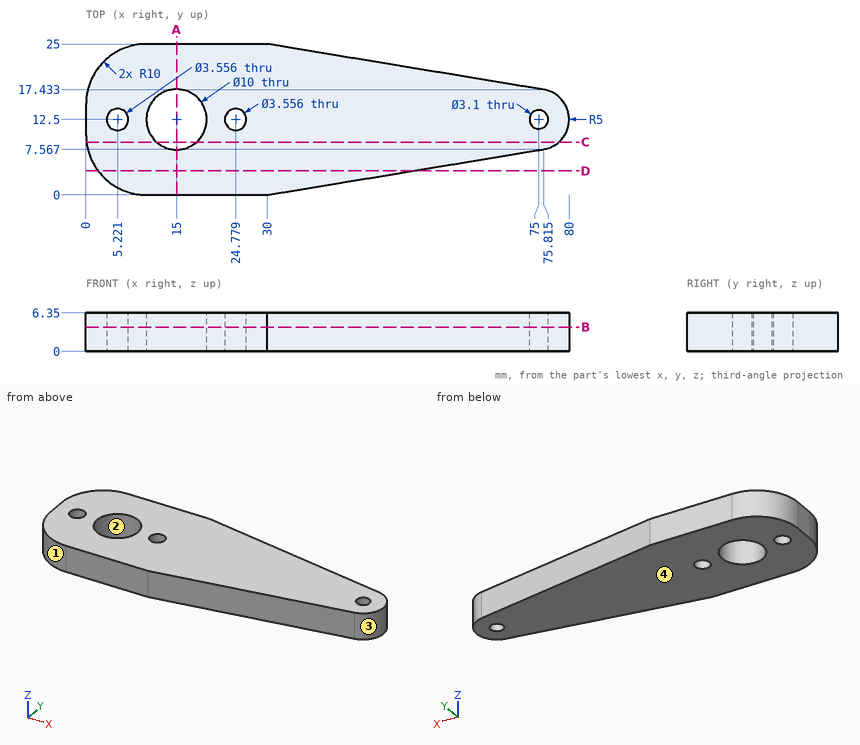
Here's the drawing with two shaded views (mm, measured from the low corner). I have some questions. Coordinates: 2 decimals unless noted, no trailing zeros. Loops run counter-clockwise (first coordinate to the right, second up) from the corner with the lowest first, then second, coordinate; pieces in that order, holes last. Notation, with made-up numbers: (77, 1.25) -> (86, 1.25) arc R16 cw to (86, 16.25) -> close; hole circle Ø6 at (-32, 69). An arc over 180 degrees is marked (long way). Answer in a Markdown table with one row per item.
(1) If I drill on probe 1 along X at (y, z) = (12.5, 2); probe 2 along X at (y, z) = (11.25, 3.5) (1 decimal); probe 3 along X at (y, z) = (8.5, 4), over which ranges is the centre line in solid material (lowest first)?
Results found:
| item | result |
|---|---|
| probe 1 | x = 0 to 3.44, 7 to 10, 20 to 23, 26.56 to 73.45, 76.55 to 80 |
| probe 2 | x = 0 to 4, 6.5 to 10.2, 19.8 to 23.5, 26 to 74.1, 75.9 to 79.8 |
| probe 3 | x = 0.11 to 12, 18 to 78 |
(2) Imagine slicing it at D-D (y = 4). List the corners of the cut face in (x, z) for me.
Results found:
| item | result |
|---|---|
| outline | (2, 0) -> (54.22, 0) -> (54.22, 6.35) -> (2, 6.35) -> close |
(3) Thinking about a two-plate mould opening in X: for the marked faces 1, 2, 3 and 4, which applies, released by +X, released by -X, zero draft, split by the parting line, or undercut?
Results found:
| item | result |
|---|---|
| face 1 | released by -X |
| face 2 | undercut |
| face 3 | released by +X |
| face 4 | zero draft |
(4) Imagine slicing it at B-B (z = 4). Give the number of separate pieces and of enclosed holes in the cut face, plus the area to 3 significant figures.
Results found:
| item | result |
|---|---|
| separate pieces | 1 |
| enclosed holes | 4 |
| area | 1,430 mm^2 |
(5) Imagine slicing it at C-C (y = 8.75). List the corners of the cut face in (x, z) for me, plus the area to 3 significant figures.
Results found:
| item | result |
|---|---|
| outline | (0.08, 0) -> (11.69, 0) -> (11.69, 6.35) -> (0.08, 6.35) -> close; (18.31, 0) -> (78.31, 0) -> (78.31, 6.35) -> (18.31, 6.35) -> close |
| area | 455 mm^2 |
(6) Will these pins go through, and if not, where does the flat tip stop? pin 1 Ø3.5 at (x, y) = (75, 12.5) entering from +Z; pin 2 Ø3 at (x, z) = (42.5, 3) entering from +Y; pin 3 Ø3 at (x, y) = (24.78, 12.5) entering from -Z.
Results found:
| item | result |
|---|---|
| pin 1 | stops at z = 6.35 |
| pin 2 | stops at y = 23.18 |
| pin 3 | passes through |
(7) Imagine slicing it at A-A (x = 15). List the corners of the cut face in (y, z) for me.
Results found:
| item | result |
|---|---|
| outline | (0, 0) -> (7.5, 0) -> (7.5, 6.35) -> (0, 6.35) -> close; (17.5, 0) -> (25, 0) -> (25, 6.35) -> (17.5, 6.35) -> close |
